CAD build for the part. Positions are in the model's coordinates, mm. Face numbers are marked on the shaded views. A direction names the side the tool comes from. Round coordinates to 2 decimals unless told otherwise and drop trailing zeros. Write each loop counter-clockwise with the first axis right and the second up, starting at its lowest first coordinate (ties: lowest second). Pieces come first, ordered by that corner, then holes. Notation, with made-up numbers: (61, -9.75) -> (93, -9.75) arc R14 ccw to (93, -5.75) -> close; hole circle Ø1 at (64, 67). An arc over 180 degrees is marked (long way). Put each result on its own line as item: value. Start each with the question number.
1. 3-axis set-ups, long thin cutter, end or side, ignore diameter. For the marked faces 1 and 2: which of +Z, -Z, +X, -X, +Y, -Y reach the whole face in a straight line?
2. Saw through at D-D on z = 39.5. List the corners of the cut face in (x, y) (3 decimals), and give its area (3 significant figures).
3. Saw through at C-C on x = 30. List the corners of the cut face in (y, z) (3 decimals), and give its area (3 significant figures).
4. Flat gauge pins, fed straight in: P1, Ø6, axis at x = 148.5, z = 17, coming from the +Y side; P2, Ø5, axis at x = 172, y = 1, coming from the -Z side; P3, Ø3, axis at x = 10.5, y = -3, coming from the -Z side. Where does each tip first touch, or does it go through?
5. Drill centre lines: line 1 (Y direction, x = 148.5, z = 32); line 2 (Z direction, x = 94, y = 1.5); line 3 (Z direction, x = 21.5, y = -3.75). Where is each one in solid material? Low to high. Write a range as from..to.
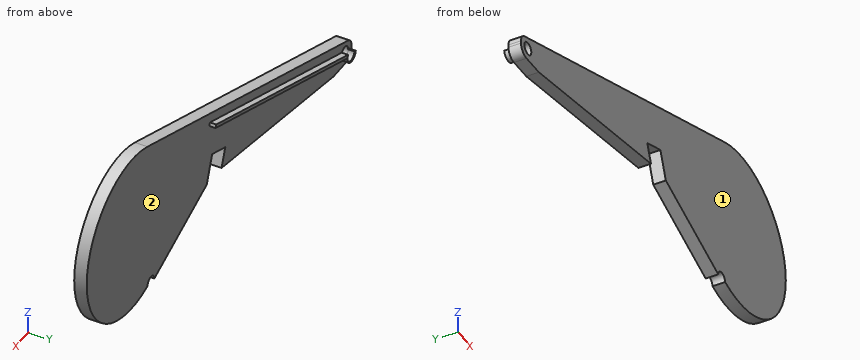
from build123d import *

# Parameters (mm, degrees)
F0_R     = 3.175
F1_DEPTH = 6.35
F2_R     = 5.08
F4_DEPTH = 3.175
F6_DEPTH = 3.175


with BuildPart() as f1:
    # F0 (on Front) → F1 (new body)
    with BuildSketch(Plane.XZ):
        with BuildLine():
            Line((0, 9.952783), (0, 0))
            Line((0, 0), (16.424974, 0))
            Line((16.424974, 0), (120.286547, 19.615395))
            Line((120.286547, 19.615395), (116.876498, 28.984427))
            Line((116.876498, 28.984427), (129.012049, 33.401406))
            Line((129.012049, 33.401406), (134.029747, 19.615395))
            Line((134.029747, 19.615395), (182.527998, 0))
            ThreePointArc((182.527998, 0), (185.702998, 3.175), (188.877998, 0))
            ThreePointArc((188.877998, 0), (245.074731, 39.349376), (188.877998, 78.698752))
            Line((188.877998, 78.698752), (0, 9.952783))
        make_face()
        with Locations((6.35, 6.35)):
            Circle(F0_R, mode=Mode.SUBTRACT)
    extrude(amount=F1_DEPTH)

    # F2
    f2_edges = [f1.edges().sort_by_distance(p)[0] for p in [
        (0, -3.175, 9.952783),
        (0, -3.175, 0),
    ]]
    fillet(f2_edges, radius=F2_R)

    # F3 (on face) → F4 (join)
    with BuildSketch(Plane(origin=(0, 0, 0), x_dir=(-1, 0, 0), z_dir=(0, 1, 0))):
        Polygon((-9.025761, 8.281487), (-131.065451, 52.700301), (-131.644688, 51.108862), (-9.604997, 6.690047), (-9.333524, 7.435914), align=None)
    extrude(amount=F4_DEPTH)

    # F5 (on face) → F6 (join)
    with BuildSketch(Plane(origin=(0, 0, 0), x_dir=(-1, 0, 0), z_dir=(0, 1, 0))):
        with BuildLine():
            Line((-9.436891, 7.151916), (-9.604997, 6.690047))
            ThreePointArc((-9.604997, 6.690047), (-6.261769, 2.230211), (-1.886095, 5.682861))
            Line((-1.886095, 5.682861), (-3.166984, 6.149066))
            ThreePointArc((-3.166984, 6.149066), (-6.853723, 3.200678), (-9.436891, 7.151916))
        make_face()
    extrude(amount=F6_DEPTH)


solid = f1.part
Return value:
1. face 1: +Z, -Z, +X, -X, -Y
1. face 2: +Y
2. outline: (81.18, -6.35) -> (245.074, -6.35) -> (245.074, 0) -> (99.75, 0) -> (99.75, 3.175) -> (94.798, 3.175) -> (94.798, 0) -> (81.18, 0) -> close
2. area: 1,060 mm^2
3. outline: (-6.35, 2.564) -> (0, 2.564) -> (0, 14.113) -> (3.175, 14.113) -> (3.175, 15.915) -> (0, 15.915) -> (0, 20.872) -> (-6.35, 20.872) -> close
3. area: 122 mm^2
4. P1: stops at y = 0
4. P2: stops at z = 3.33
4. P3: stops at z = 0
5. line 1: y = -6.35..0
5. line 2: z = 37.41..39.21
5. line 3: z = 0.96..17.78
